For this review, take the finished solid that the model builds, in its own axes (mm). A direction names the side the tool comes from. Round coordinates to 2 decimals unless told otherwise and drop trailing zeros. Order: outer loops, then holes, each group sorted by start corner. A loop starts at its lowest first (then second) coordinate and runs counter-clockwise, first axis right, second up. Notation, with made-up numbers: M 3,82 L 10,82 A12 cw 10,93 Z; hole C -15,-29 d10. An arc over 180 degrees is marked long. Answer in a Markdown table with one row per item. Add a question column.
```python
from build123d import *

# Parameters (mm, degrees)
SKETCH2_R           = 11.125
BOSS_EXTRUDE1_DEPTH = 8
SKETCH3_R           = 10
BOSS_EXTRUDE2_DEPTH = 2
BOSS_EXTRUDE3_DEPTH = 75
CUT_EXTRUDE1_DEPTH  = 85.433405711
BOSS_EXTRUDE4_DEPTH = 1.34
CUT_EXTRUDE4_DEPTH  = 81.030594237
SKETCH14_R          = 1.5
CUT_EXTRUDE6_DEPTH  = 10


with BuildPart() as part:
    # Sketch2 → Boss-Extrude1 (new body)
    with BuildSketch(Plane(origin=(0, 0, 0), x_dir=(1, 0, 0), z_dir=(0, 1, 0))):
        Polygon((0, 17.320508076), (-15, 8.660254038), (-15, -8.660254038), (0, -17.320508076), (15, -8.660254038), (15, 8.660254038), align=None)
        with Locations(Location((0, 0, 0), (0, 0, 270))):
            Circle(SKETCH2_R, mode=Mode.SUBTRACT)
    extrude(amount=BOSS_EXTRUDE1_DEPTH)

    # Sketch3 → Boss-Extrude2 (add)
    with BuildSketch(Plane.XZ):
        Polygon((0, 17.320508076), (-15, 8.660254038), (-15, -8.660254038), (0, -17.320508076), (15, -8.660254038), (15, 8.660254038), align=None)
        with Locations(Location((0, 0, 0), (0, 0, 270))):
            Circle(SKETCH3_R, mode=Mode.SUBTRACT)
    extrude(amount=BOSS_EXTRUDE2_DEPTH)

    # Sketch4 → Boss-Extrude3 (add)
    with BuildSketch(Plane.XZ.offset(2)):
        Polygon((-10, 11.547005384), (-15, 8.660254038), (-15, -8.660254038), (-10, -11.547005384), align=None)
        Polygon((10, -11.547005384), (15, -8.660254038), (15, 8.660254038), (10, 11.547005384), align=None)
    extrude(amount=BOSS_EXTRUDE3_DEPTH)

    # Sketch5 → Cut-Extrude1 (cut, through all)
    with BuildSketch(Plane.ZY.offset(15)):
        Polygon((11.547005384, -77), (-11.547005384, -63.666666667), (-11.547005384, -77), align=None)
    extrude(amount=-CUT_EXTRUDE1_DEPTH, mode=Mode.SUBTRACT)

    # Sketch6 → Boss-Extrude4 (add)
    with BuildSketch(Plane(origin=(0, -52.75, -30.4552267), x_dir=(1, 0, 0), z_dir=(-1.6525460586108427e-15, -0.8660254037844438, -0.4999999999999913))):
        Polygon((-10, 48.5), (-15, 45.166666667), (-15, 25.166666667), (-10, 21.833333333), align=None)
        Polygon((10, 48.5), (15, 45.166666667), (15, 25.166666667), (10, 21.833333333), align=None)
    extrude(amount=BOSS_EXTRUDE4_DEPTH)

    # Sketch9 → Cut-Extrude4 (cut, through all)
    with BuildSketch(Plane(origin=(0, -53.910474041, -31.1252267), x_dir=(1, 0, 0), z_dir=(0, -0.8660254037844435, -0.4999999999999916))):
        Polygon((-15, 45.166666667), (-10, 38.5), (-10, 48.5), align=None)
        Polygon((10, 48.5), (10, 38.5), (15, 45.166666667), align=None)
    extrude(amount=-CUT_EXTRUDE4_DEPTH, mode=Mode.SUBTRACT)

    # Sketch14 → Cut-Extrude6 (cut)
    with BuildSketch(Plane(origin=(0, -53.910474041, -31.1252267), x_dir=(1, 0, 0), z_dir=(-3.0355825822191097e-15, -0.8660254037844435, -0.4999999999999916))):
        with Locations(Location((-12.498602075, 34.732241333, 0), (0, 0, 270))):
            Circle(SKETCH14_R)
        with Locations(Location((-12.498602075, 27.580286063, 0), (0, 0, 270))):
            Circle(SKETCH14_R)
        with Locations(Location((12.498602075, 27.580286063, 0), (0, 0, 270))):
            Circle(SKETCH14_R)
        with Locations(Location((12.498602075, 37.148097384, 0), (0, 0, 270))):
            Circle(SKETCH14_R)
    extrude(amount=-CUT_EXTRUDE6_DEPTH, mode=Mode.SUBTRACT)


solid = part.part
```
1. Clearance check with flat-ended pins moving along their axes: pin 1 Ø14 at (x, z) = (0, 10) entering from -Y; pin 2 Ø2 at (y, z) = (-53.5, 11) entering from -X. State where each tip first meets the part, or that it passes through.
2. Consider section D-D on x = -5.5. Write out the cut boundary in (y, z), plus the area to 3 significant figures.
3. The part is to be moulded in two halves that separate along Y. For faces 1 (the flat face through (12.535, -70.742, -1.972)), 2 (the flat face through (10.938, -23.824, 11.005)), 3 (the cylindrical face through (-13.07, -66.31, 0.22)), 4 (the cylindrical face through (12, -68, 2)), say which applies: pulls with the +Y half, pulls with the -Y half, needs draft (parallel to the pull), parting line crosses it, or undercut.
4. Consider section B-B on x = 4. Write out the cut boundary in (y, z), plus the area to 3 significant figures.
5. Consider section C-C on y = -6.5. Write out the cut boundary in (x, z), plus the area to 3 significant figures.
6. For faces 5 (the flat face through (12.52, -63.835, 6.064)), 6 (the cylindrical face through (7.52, 3.94, -8.2)), 7 (the flat face through (10, -37, 0)), 8 (the flat face through (11.909, -68.262, 7.985)), 9 (the flat face through (-10.938, -20.005, -11.005)), list the 3-axis set-ups (+Z, -Z, +X, -X, +Y, -Y) from which the entire face can be reached by the end or side of a thin tool; tool diameter is ignored.
7. To check wall thickness, follow probe 1 along X at (y, z) = (-59, 7); probe 2 along Z at (x, y) = (0, -0.8); probe 3 along Y at (x, z) = (7.5, 12.5). State the ranges of each line that lie inside material, in increasing order. Write a range as [from, to].
Solved:
| question | item | result |
|---|---|---|
| 1 | pin 1 | stops at y = -2 |
| 1 | pin 2 | stops at x = -12.68 |
| 2 | outline | M -2,-14.15 L 8,-14.15 L 8,-9.67 L 0,-9.67 L 0,-8.35 L -2,-8.35 Z; M -2,8.35 L 0,8.35 L 0,9.67 L 8,9.67 L 8,14.15 L -2,14.15 Z |
| 2 | area | 94.8 mm^2 |
| 3 | face 1 | pulls with the -Y half |
| 3 | face 2 | needs draft |
| 3 | face 3 | undercut |
| 3 | face 4 | undercut |
| 4 | outline | M -2,-15.01 L 8,-15.01 L 8,-10.38 L 0,-10.38 L 0,-9.17 L -2,-9.17 Z; M -2,9.17 L 0,9.17 L 0,10.38 L 8,10.38 L 8,15.01 L -2,15.01 Z |
| 4 | area | 97.5 mm^2 |
| 5 | outline | M -15,-8.66 L -10,-11.55 L -10,11.55 L -15,8.66 Z; M 10,-11.55 L 15,-8.66 L 15,8.66 L 10,11.55 Z |
| 5 | area | 202 mm^2 |
| 6 | face 5 | none |
| 6 | face 6 | +Y |
| 6 | face 7 | +Z, -Z, -Y |
| 6 | face 8 | +Z, -Y |
| 6 | face 9 | -Z, -X, +Y |
| 7 | probe 1 | x = [-15, -10], [10, 15] |
| 7 | probe 2 | z = [-17.32, -10], [10, 17.32] |
| 7 | probe 3 | y = [-2, 8] |
